Here's how the part is built. I have some questions about the finished solid (model axes, mm). Face numbers are marked on the shaded views. A direction names the side the tool comes from. Give positions to 0.01 mm unless a question says otherwise; leave off trailing zeros. Write each loop counter-clockwise with the first axis right and the second up, starting at its lowest first coordinate (ties: lowest second). Pieces come first, ordered by that corner, then holes. Notation, with made-up numbers: (-33, -21.75) - (10, -21.75) arc R20 cw to (10, 3.25) - close; hole circle Ø7 at (-36.75, -36.5). An arc over 180 degrees is marked (long way). One line per item, written item: value. Start each with the question number.
1) Please list where these lines run through material, in increasing order: L1, parallel to X at y = 1.6, z = 8.5; L2, parallel to X at y = 0.7, z = 1; L3, parallel to Y at x = 15, z = 11.25. Write a range as [from, to].
2) I'm going to push flat-ended pins straight in: P1, Ø0.7, axis at x = 34.5, y = 2, coming from the -Z side; P2, Ø2.5, axis at x = 14, z = 12.5, coming from the -Y side. Where does each tip first touch, or does it pass through?
3) Imagine slicing it at A-A on y = 1.15. Count the separate pieces of the cut face and the enclosed holes in it, plus the area to 3 significant figures.
4) We'd pull the mould along Z, two halves only. Please class the marked faces 4, 5 and 6: +Z half, -Z half, draft (parallel to the pull), parting line (faces both ways), or undercut.
5) Imagine slicing it at D-D on y = 3.9. Write out the boundary of the cut face in (x, z), plus the area to 3 significant figures.
6) Imagine slicing it at B-B on z = 7.75. Write out the boundary of the cut face in (x, y).
7) On a 3-axis mill with a long thin cutter (end or side, diameter ignored), from which of +Z, -Z, +X, -X, +Y, -Y can I reach the whole of each face in a straight line? I mean the marked faces 1, 2 and 3. Say none if no direction works.
8) Imagine slicing it at C-C on x = 18. Write out the boundary of the cut face in (y, z), plus the area to 3 significant figures.
from build123d import *

# Parameters (mm, degrees)
SKETCH1_W               = 37.29
SKETCH1_H               = 4.5
BOSS_EXTRUDE1_DEPTH     = 20
CUT_EXTRUDE1_DEPTH      = 43.553426419
CUT_EXTRUDE1_DEPTH_BACK = 43.553426419
SKETCH1_3_W             = 3.1
SKETCH1_3_H             = 3
CUT_EXTRUDE2_START      = 9
SKETCH1_4_W             = 4.85
SKETCH1_4_H             = 3
CUT_EXTRUDE2_DEPTH      = 5.5
SKETCH1_5_W             = 5
SKETCH1_5_H             = 3.5
CUT_EXTRUDE3_DEPTH      = 2.5
FILLET1_R               = 3


with BuildPart() as part:
    # Sketch1 → Boss-Extrude1 (new body)
    with BuildSketch(Plane.XY):
        with Locations((18.645, 2.25)):
            Rectangle(SKETCH1_W, SKETCH1_H)
    extrude(amount=BOSS_EXTRUDE1_DEPTH)

    # Sketch1<3> → Cut-Extrude1 (cut, two sides: drawn at the far end of the back side and taken through both)
    with BuildSketch(Plane.XY.offset(-CUT_EXTRUDE1_DEPTH_BACK)):
        with Locations((4.5, 1.5)):
            Rectangle(SKETCH1_3_W, SKETCH1_3_H)
        with Locations((13.93, 1.5)):
            Rectangle(SKETCH1_3_W, SKETCH1_3_H)
        with Locations((23.36, 1.5)):
            Rectangle(SKETCH1_3_W, SKETCH1_3_H)
        with Locations((32.79, 1.5)):
            Rectangle(SKETCH1_3_W, SKETCH1_3_H)
    extrude(amount=CUT_EXTRUDE1_DEPTH + CUT_EXTRUDE1_DEPTH_BACK, mode=Mode.SUBTRACT)

    # Sketch1<4> → Cut-Extrude2 (cut)
    with BuildSketch(Plane.XY.offset(CUT_EXTRUDE2_START)):
        with Locations((4.5, 1.5)):
            Rectangle(SKETCH1_4_W, SKETCH1_4_H)
        with Locations((13.93, 1.5)):
            Rectangle(SKETCH1_4_W, SKETCH1_4_H)
        with Locations((23.36, 1.5)):
            Rectangle(SKETCH1_4_W, SKETCH1_4_H)
        with Locations((32.79, 1.5)):
            Rectangle(SKETCH1_4_W, SKETCH1_4_H)
    extrude(amount=CUT_EXTRUDE2_DEPTH, mode=Mode.SUBTRACT)

    # Sketch1<5> → Cut-Extrude3 (cut)
    with BuildSketch(Plane.XY):
        with Locations((4.5, 1.75)):
            Rectangle(SKETCH1_5_W, SKETCH1_5_H)
        with Locations((13.93, 1.75)):
            Rectangle(SKETCH1_5_W, SKETCH1_5_H)
        with Locations((23.36, 1.75)):
            Rectangle(SKETCH1_5_W, SKETCH1_5_H)
        with Locations((32.79, 1.75)):
            Rectangle(SKETCH1_5_W, SKETCH1_5_H)
    extrude(amount=CUT_EXTRUDE3_DEPTH, mode=Mode.SUBTRACT)

    # Fillet1
    # the kernel refuses this fillet: 3 mm, written as the material it takes off along each edge
    with BuildSketch(Plane(origin=(-7.5, 4.5, 20), x_dir=(0, 0, -1), z_dir=(1, 0, 0))) as fillet1_piece_1:
        with BuildLine():
            CenterArc((FILLET1_R, -FILLET1_R), FILLET1_R, 90, 90)
            Line((0, -FILLET1_R), (0, 0))
            Line((0, 0), (FILLET1_R, 0))
        make_face()
    extrude(amount=52.29, mode=Mode.SUBTRACT)
    with BuildSketch(Plane(origin=(37.29, 4.5, -7.5), x_dir=(-1, 0, 0), z_dir=(0, 0, 1)), Plane(origin=(0, 4.5, -7.5), x_dir=(0, -1, 0), z_dir=(0, 0, 1))) as fillet1_piece_2:
        with BuildLine():
            CenterArc((FILLET1_R, FILLET1_R), FILLET1_R, 180, 90)
            Line((0, FILLET1_R), (0, 0))
            Line((0, 0), (FILLET1_R, 0))
        make_face()
    extrude(amount=35, mode=Mode.SUBTRACT)


solid = part.part
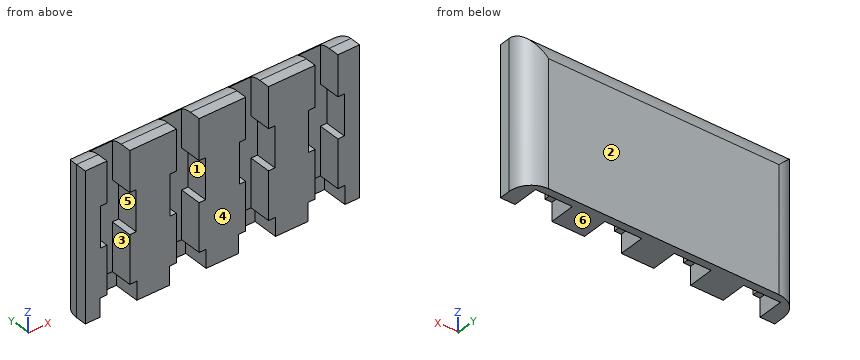
Numbers:
1. L1: [0, 2.95], [6.05, 12.38], [15.48, 21.81], [24.91, 31.24], [34.34, 37.29]
1. L2: [0, 2], [7, 11.43], [16.43, 20.86], [25.86, 30.29], [35.29, 37.29]
1. L3: [3, 4.5]
2. P1: z = 2.5
2. P2: y = 3
3. separate pieces: 5
3. enclosed holes: 0
3. area: 440 mm^2
4. face 4: draft
4. face 5: undercut
4. face 6: -Z half
5. outline: (1.2, 0) - (36.09, 0) - (36.09, 18.8) - (1.2, 18.8) - close
5. area: 656 mm^2
6. outline: (0, 0) - (2.95, 0) - (2.95, 3) - (6.05, 3) - (6.05, 0) - (12.38, 0) - (12.38, 3) - (15.48, 3) - (15.48, 0) - (21.81, 0) - (21.81, 3) - (24.91, 3) - (24.91, 0) - (31.24, 0) - (31.24, 3) - (34.34, 3) - (34.34, 0) - (37.29, 0) - (37.29, 1.5) arc R3 ccw to (34.29, 4.5) - (3, 4.5) arc R3 ccw to (0, 1.5) - close
7. face 1: -Y
7. face 2: +Z, -Z, +X, -X, +Y
7. face 3: +Z, -Z, -Y
8. outline: (0, 0) - (4.5, 0) - (4.5, 17) arc R3 ccw to (1.5, 20) - (0, 20) - close
8. area: 88.1 mm^2
